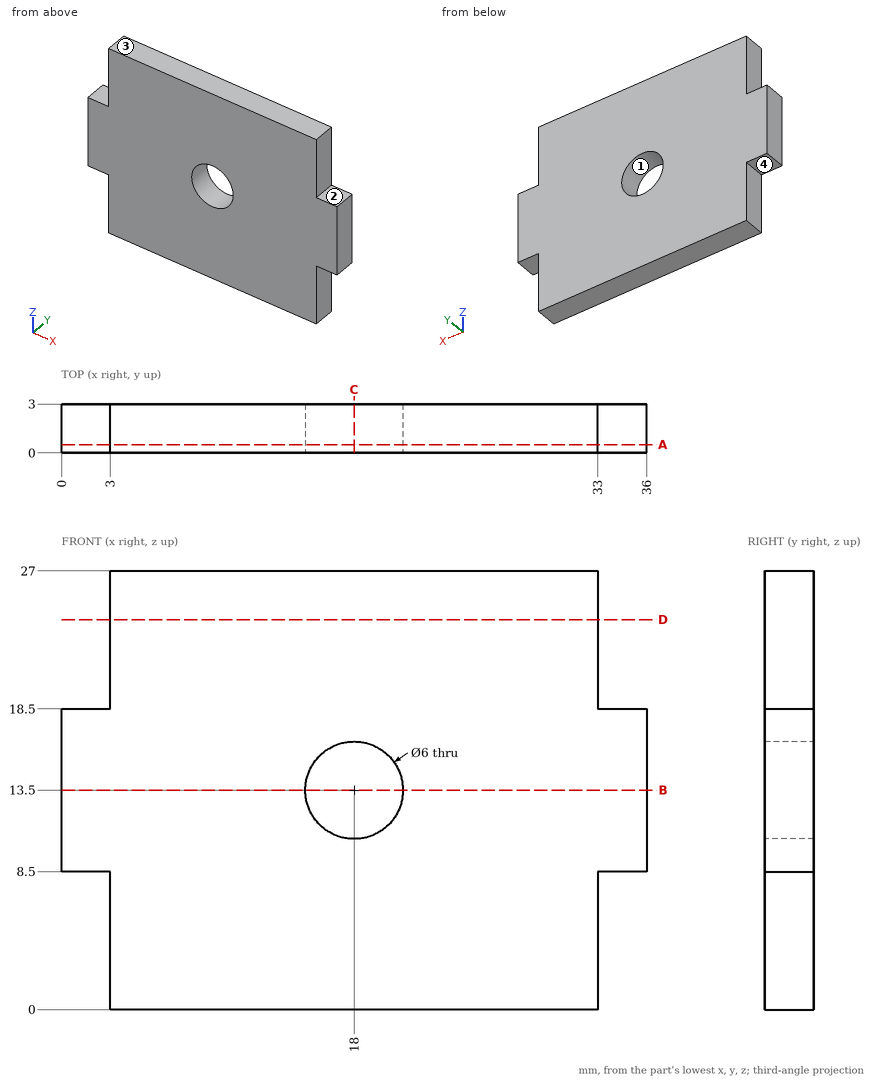
Source: three-view drawing plus pictorial views. Frame: mm from the lowest corner of the part. A direction names the side the tool comes from. Coordinates: 2 decimals unless noted, no trailing zeros. Order: outer loops, then holes, each group sorted by start corner. A loop starts at its lowest first (then second) coordinate and runs counter-clockwise, first axis right, second up. Notation, with made-up numbers: (72, -37.5) -> (98, -37.5) arc R37 cw to (98, -0.5) -> close; hole circle Ø10 at (75, 61.25). An arc over 180 degrees is marked (long way). Write item = value, one per line.
(1) Pin query (flat end, axial travel): pin 1 Ø1.5 at (x, y) = (1, 2) entering from +Z; pin 2 Ø4 at (x, z) = (18.5, 13) entering from +Y; pin 3 Ø0.9 at (x, y) = (1.5, 1.5) entering from -Z; pin 4 Ø0.9 at (y, z) = (1.5, 22) entering from +X. Return the tip coordinate at first contact, or that it passes through.
Solved:
pin_1 = 18.5
pin_2 = through
pin_3 = 8.5
pin_4 = 33
(2) Access query for the marked faces 3 and 4. Directions: +Z, -Z, +X, -X, +Y, -Y. A direction counts if a zero-diameter tool reaches every point of the face in a straight line with its end or side. Return the directions, or none.
Solved:
face_3 = +Z, +X, -X, +Y, -Y
face_4 = -Z, -X, +Y, -Y
(3) Cut plane C-C on x = 18. Return loops of the section in (y, z), plus the area to 3 significant figures.
Solved:
outline = (0, 0) -> (3, 0) -> (3, 10.5) -> (0, 10.5) -> close; (0, 16.5) -> (3, 16.5) -> (3, 27) -> (0, 27) -> close
area = 63.0 mm²
(4) Cut plane A-A on y = 0.5. Return loops of the section in (x, z).
Solved:
outline = (0, 8.5) -> (3, 8.5) -> (3, 0) -> (33, 0) -> (33, 8.5) -> (36, 8.5) -> (36, 18.5) -> (33, 18.5) -> (33, 27) -> (3, 27) -> (3, 18.5) -> (0, 18.5) -> close; hole circle Ø6 at (18, 13.5)
(5) Cut plane D-D on z = 24. Return loops of the section in (x, y), plus the area to 3 significant figures.
Solved:
outline = (3, 0) -> (33, 0) -> (33, 3) -> (3, 3) -> close
area = 90.0 mm²
(6) Pull-direction query (X, two-part tool) for the marked faces 1 and 2; classes: pulls with the +X half, pulls with the -X half, needs draft (parallel to the pull), parting line crosses it, or undercut.
Solved:
face_1 = undercut
face_2 = needs draft
(7) Line query: line 1 (X direction, y = 1.55, z = 13.5); line 2 (Z direction, x = 33.5, y = 1.45); line 3 (X direction, y = 1.5, z = 2.25). Output: solid intervals per line, ascending.
Solved:
line_1 = 0 to 15, 21 to 36
line_2 = 8.5 to 18.5
line_3 = 3 to 33
(8) Cut plane B-B on z = 13.5. Return loops of the section in (x, y).
Solved:
outline = (0, 0) -> (15, 0) -> (15, 3) -> (0, 3) -> close; (21, 0) -> (36, 0) -> (36, 3) -> (21, 3) -> close
